Build history of the part. All positions in model axes, mm. Face numbers are marked on the shaded views. A direction names the side the tool comes from. Give positions to 0.01 mm unless a question says otherwise; leave off trailing zeros. Write each loop counter-clockwise with the first axis right and the second up, starting at its lowest first coordinate (ties: lowest second). Pieces come first, ordered by that corner, then holes. Notation, with made-up numbers: (3.25, 82) -> (46.25, 82) arc R6 cw to (46.25, 92) -> close; hole circle Ø1 at (8, 71.5). An arc over 180 degrees is marked (long way). Write item = value, one per line. Start each with the question number.
Q1. Saw through at B-B, the plane y = -30. List the corners of the cut face in (x, z).
Q2. Tool access for the marked faces 4 and 5: list every direction of +Z, -Z, +X, -X, +Y, -Y with a clear straight run to the whole face (end or side of a thin tool).
Q3. Saw through at C-C, the plane z = -7.5. List the corners of the cut face in (x, y).
Q4. Wall check: line 1 (Y direction, x = 0, z = 2.75); line 2 (X direction, y = -22, z = -36); line 3 (Y direction, x = -27.5, z = -7.5). Give the ranges that are in metal, low to high.
Q5. Mould opens along X. For the marked faces 1, 2 and 3 say: pulls with the +X half, pulls with the -X half, needs draft (parallel to the pull), parting line crosses it, or undercut.
Q6. Drop flat-ended pins along their axis: P1, Ø1.2, axis at y = -33, z = -51.5, coming from the +X side; P2, Ø1.5, axis at x = 19.5, y = 5, coming from the -Z side; P3, Ø2, axis at x = 27, y = 0, coming from the -Z side; P4, Ø1.5, axis at x = -27, z = -52.5, coming from the +Y side. Give the stop position or say it passes through.
Q7. Saw through at A-A, the plane x = 0. List the corners of the cut face in (y, z), then the cut area to 3 significant figures.
Q8. Saw through at D-D, the plane z = -46.5. List the corners of the cut face in (x, y), then the cut area to 3 significant figures.
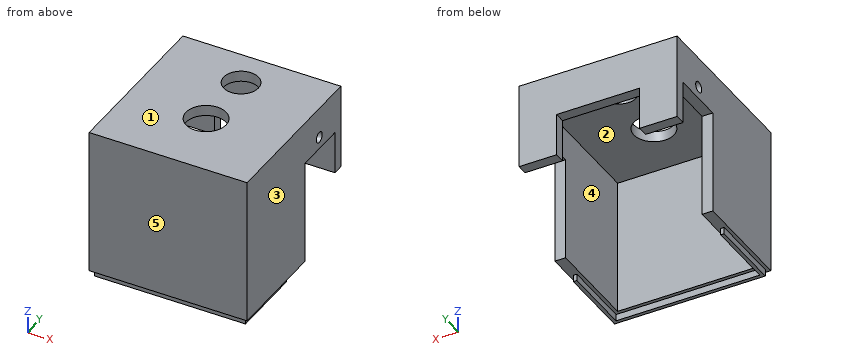
from build123d import *

# Parameters (mm, degrees)
SKETCH1_W           = 59
SKETCH1_H           = 20
SKETCH1_R           = 6.5
BOSS_EXTRUDE1_DEPTH = 4
SKETCH2_W           = 59
SKETCH2_H           = 16
BOSS_EXTRUDE2_DEPTH = 4
SKETCH3_W           = 14
SKETCH3_H           = 4
BOSS_EXTRUDE3_DEPTH = 16
SKETCH4_W           = 4
SKETCH4_H           = 20
BOSS_EXTRUDE4_DEPTH = 12
SKETCH5_R           = 2
CUT_EXTRUDE1_DEPTH  = 80
BOSS_EXTRUDE7_DEPTH = 35
SKETCH9_W           = 59
SKETCH9_H           = 55
BOSS_EXTRUDE8_DEPTH = 4
SKETCH10_W          = 55
SKETCH10_H          = 1.333333334
SKETCH10_W_2        = 1.333333334
SKETCH10_H_2        = 26.333333333
BOSS_EXTRUDE9_DEPTH = 2.5
SKETCH11_R          = 7.5
CUT_EXTRUDE2_DEPTH  = 5


with BuildPart() as part:
    # Sketch1 → Boss-Extrude1 (new body)
    with BuildSketch(Plane.XY):
        Rectangle(SKETCH1_W, SKETCH1_H)
        Circle(SKETCH1_R, mode=Mode.SUBTRACT)
    extrude(amount=BOSS_EXTRUDE1_DEPTH)

    # Sketch2 → Boss-Extrude2 (add)
    with BuildSketch(Plane(origin=(0, 10, 0), x_dir=(1, 0, 0), z_dir=(0, 1, 0))):
        with Locations((0, 4)):
            Rectangle(SKETCH2_W, SKETCH2_H)
    extrude(amount=BOSS_EXTRUDE2_DEPTH)

    # Sketch3 → Boss-Extrude3 (add)
    with BuildSketch(Plane(origin=(0, 0, -12), x_dir=(-1, 0, 0), z_dir=(0, 0, -1))):
        with Locations((-22.5, 12)):
            Rectangle(SKETCH3_W, SKETCH3_H)
        with Locations((22.5, 12)):
            Rectangle(SKETCH3_W, SKETCH3_H)
    extrude(amount=BOSS_EXTRUDE3_DEPTH)

    # Sketch4 → Boss-Extrude4 (add)
    with BuildSketch(Plane(origin=(0, 0, 0), x_dir=(-1, 0, 0), z_dir=(0, 0, -1))):
        with Locations((27.5, 0)):
            Rectangle(SKETCH4_W, SKETCH4_H)
        with Locations((-27.5, 0)):
            Rectangle(SKETCH4_W, SKETCH4_H)
    extrude(amount=BOSS_EXTRUDE4_DEPTH)

    # Sketch5 → Cut-Extrude1 (cut)
    with BuildSketch(Plane.ZY.offset(29.5)):
        with Locations((-7.5, -0.5)):
            Circle(SKETCH5_R)
    extrude(amount=-CUT_EXTRUDE1_DEPTH, mode=Mode.SUBTRACT)

    # Sketch8 → Boss-Extrude7 (add)
    with BuildSketch(Plane.XZ.offset(10)):
        Polygon((25.5, -51), (29.5, -51), (29.5, 4), (-29.5, 4), (-29.5, -51), (-25.5, -51), (-25.5, 0), (25.5, 0), align=None)
    extrude(amount=BOSS_EXTRUDE7_DEPTH)

    # Sketch9 → Boss-Extrude8 (add)
    with BuildSketch(Plane.XZ.offset(45)):
        with Locations((0, -23.5)):
            Rectangle(SKETCH9_W, SKETCH9_H)
    extrude(amount=BOSS_EXTRUDE8_DEPTH)

    # Sketch10 → Boss-Extrude9 (add)
    with BuildSketch(Plane(origin=(0, 0, -51), x_dir=(-1, 0, 0), z_dir=(0, 0, -1))):
        Polygon((-28.166666667, -47.666666667), (-26.833333333, -47.666666667), (-26.833333333, -46.333333333), (-26.833333333, -20), (-28.166666667, -20), align=None)
        with Locations((0.666666667, -47)):
            Rectangle(SKETCH10_W, SKETCH10_H)
        with Locations((27.5, -33.166666667)):
            Rectangle(SKETCH10_W_2, SKETCH10_H_2)
    extrude(amount=BOSS_EXTRUDE9_DEPTH)

    # Sketch11 → Cut-Extrude2 (cut)
    with BuildSketch(Plane.XY.offset(4)):
        with Locations((0, -23.5)):
            Circle(SKETCH11_R)
    extrude(amount=-CUT_EXTRUDE2_DEPTH, mode=Mode.SUBTRACT)


solid = part.part
Report:
q1.outline = (-29.5, -51) -> (-28.17, -51) -> (-28.17, -53.5) -> (-26.83, -53.5) -> (-26.83, -51) -> (-25.5, -51) -> (-25.5, 0) -> (-3.74, 0) -> (-3.74, 4) -> (-29.5, 4) -> close; (3.74, 0) -> (25.5, 0) -> (25.5, -51) -> (26.83, -51) -> (26.83, -53.5) -> (28.17, -53.5) -> (28.17, -51) -> (29.5, -51) -> (29.5, 4) -> (3.74, 4) -> close
q2.face_4 = -Z
q2.face_5 = +Z, -Z, +X, -X, -Y
q3.outline = (-29.5, -49) -> (29.5, -49) -> (29.5, -2.5) -> (25.5, -2.5) -> (25.5, -45) -> (-25.5, -45) -> (-25.5, -2.5) -> (-29.5, -2.5) -> close; (-29.5, 1.5) -> (-25.5, 1.5) -> (-25.5, 10) -> (25.5, 10) -> (25.5, 1.5) -> (29.5, 1.5) -> (29.5, 14) -> (-29.5, 14) -> close
q4.line_1 = -49 to -31, -16 to -6.5, 6.5 to 14
q4.line_2 = -29.5 to -25.5, 25.5 to 29.5
q4.line_3 = -49 to -2.5, 1.5 to 14
q5.face_1 = needs draft
q5.face_2 = undercut
q5.face_3 = pulls with the +X half
q6.P1 = 29.5
q6.P2 = 0
q6.P3 = -12
q6.P4 = -20
q7.outline = (-49, -51) -> (-47.67, -51) -> (-47.67, -53.5) -> (-46.33, -53.5) -> (-46.33, -51) -> (-45, -51) -> (-45, 0) -> (-31, 0) -> (-31, 4) -> (-49, 4) -> close; (-16, 0) -> (-6.5, 0) -> (-6.5, 4) -> (-16, 4) -> close; (6.5, 0) -> (10, 0) -> (10, -12) -> (14, -12) -> (14, 4) -> (6.5, 4) -> close
q7.area = 395 mm2
q8.outline = (-29.5, -49) -> (29.5, -49) -> (29.5, -10) -> (25.5, -10) -> (25.5, -45) -> (-25.5, -45) -> (-25.5, -10) -> (-29.5, -10) -> close
q8.area = 516 mm2
